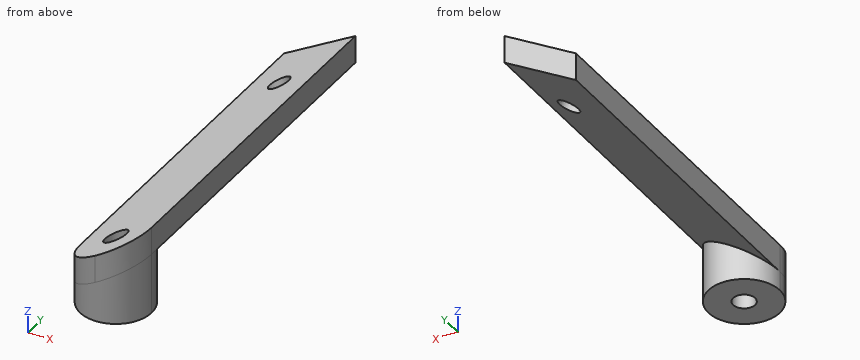
Autodesk Inventor part; units mm, degrees
ref_plane "YZ Plane" through (0, 0, 0) normal (1, 0, 0) x (0, 1, 0)
ref_plane "XZ Plane" through (0, 0, 0) normal (0, 1, 0) x (-1, 0, 0)
ref_plane "XY Plane" through (0, 0, 0) normal (0, 0, 1) x (1, 0, 0)
sketch "Sketch1" plane through (0, 0, 0) normal (0, 1, 0) x (-1, 0, 0)
  line L0 (0, 14.6647) -> (-13, 22.1703)
  line L1 (0, 14.6647) -> (15.0111, 14.6647) construction
  line L2 (-13, 22.1703) -> (-13, 27.1703)
  line L3 (0, 19.6647) -> (0, 14.6647)
  line L4 (0, 0) -> (-28.4468, 0) construction
  line L5 (-13, -7.1591) -> (0, -14.6647)
  line L6 (0, -14.6647) -> (0, -19.6647)
  line L7 (-13, 27.1703) -> (0, 27.1703)
  line L8 (0, 27.1703) -> (0, 19.6647)
  line L9 (0, -19.6647) -> (-13, -19.6647)
  line L10 (-13, -19.6647) -> (-13, -7.1591)
  point P0 (0, -12.7)
  dimension "d1" = 150
  dimension "d2" = 5
  dimension "d5" = 25.4
  dimension "d6" = 0
  dimension "d7" = 0
  dimension "d8" = 14.6647
  dimension "d9" = 13
  dimension "d10" = 13
  dimension "d11" = 5
extrude "Extrusion1" add sketch "Sketch1" against normal blind 70.4
fillet "Fillet1" radius 6.5 4 edges at (0, -70.4, 20.9175) (13, -70.4, 24.6703) (13, -70.4, -13.4119) (0, -70.4, -17.1647)
sketch "Sketch2" plane through (0, 0, 27.1703) normal (0, 0, 1) x (1, 0, 0)
  arc A0 (0, -63.9) -> (13, -63.9) centre (6.5, -63.9) ccw
  line L0 (0, -63.9) -> (0, 0)
  line L1 (0, 0) -> (13, 0)
  line L2 (13, 0) -> (13, -63.9)
  circle A1 centre (6.5, -63.9) radius 6.5
extrude "Extrusion2" add sketch "Sketch2" against normal blind 16 contours A1 A0
sketch "Sketch3" plane through (13, 0, -19.6647) normal (0, 0, -1) x (-1, 0, 0)
  arc A0 (0, -63.9) -> (13, -63.9) centre (6.5, -63.9) ccw
  line L0 (0, -63.9) -> (0, 0)
  line L1 (0, 0) -> (13, 0)
  line L2 (13, 0) -> (13, -63.9)
  circle A1 centre (6.5, -63.9) radius 6.5
extrude "Extrusion3" add sketch "Sketch3" against normal blind 16 contours A1 A0
sketch "Sketch4" plane through (0, 0, 0) normal (0, 1, 0) x (1, 0, 0)
  line L0 (0, -14.6647) -> (13, -22.1703)
  line L1 (13, -22.1703) -> (13, -27.1703)
  line L2 (13, -27.1703) -> (0, -27.1703)
  line L3 (0, -27.1703) -> (0, -14.6647)
  line L4 (13, 7.1591) -> (0, 14.6647)
  line L5 (0, 14.6647) -> (0, 19.6647)
  line L6 (0, 19.6647) -> (13, 19.6647)
  line L7 (13, 19.6647) -> (13, 7.1591)
  line L8 (13, -27.1703) -> (0, -19.6647)
  line L9 (13, -27.1703) -> (28.0111, -27.1703) construction
  line L10 (0, 19.6647) -> (13, 12.1591)
  point P0 (0, 0)
  dimension "d19" = 150
extrude "Extrusion4" cut sketch "Sketch4" against normal through all contours L8 L2 L3 | L10 L6 L7
sketch "Sketch5" plane through (13, -63.9, 27.1703) normal (-0.5, 0, 0.8660254) x (0.8660254, 0, 0.5)
  ellipse E0 centre (-7.5056, 0) end of major axis (-15.0111, 0) minor radius 6.5 (-15.0111, 0) -> (0, 0) ccw
  line L0 (-15.0111, 0) -> (-15.0111, 63.9)
  line L1 (-15.0111, 63.9) -> (0, 63.9)
  line L2 (0, 63.9) -> (0, 0)
  circle A0 centre (-7.5056, 51.2) radius 2
  point P0 (-24.8435, 63.9)
  dimension "d22" = 4
  dimension "d23" = 12.7
extrude "Extrusion5" cut sketch "Sketch5" against normal up to next contours A0
sketch "Sketch6" plane through (0, -63.9, -19.6647) normal (0.5, 0, -0.8660254) x (-0.8660254, 0, -0.5)
  ellipse E0 centre (-7.5056, 0) end of major axis (-15.0111, 0) minor radius 6.5 (-15.0111, 0) -> (0, 0) ccw
  line L0 (-15.0111, 0) -> (-15.0111, 63.9)
  line L1 (-15.0111, 63.9) -> (0, 63.9)
  line L2 (0, 63.9) -> (0, 0)
  circle A0 centre (-7.5056, 51.2) radius 2
  point P0 (-9.8323, 63.9)
  dimension "d26" = 4
  dimension "d27" = 12.7
extrude "Extrusion6" cut sketch "Sketch6" against normal up to next contours A0
sketch "Sketch7" plane through (6.5, -63.9, -3.6647) normal (0, 0, 1) x (1, 0, 0)
  circle A0 centre (0, 0) radius 6.5
  circle A1 centre (0, 0) radius 2
  point P0 (-6.5, 63.9)
  dimension "d30" = 4
extrude "Extrusion7" cut sketch "Sketch7" along normal through all both and the other way through all contours A1
sketch "Sketch9" plane through (0, 0, 0) normal (0, 1, 0) x (1, 0, 0)
  line L0 (-2.3389, 1.3365) -> (18.6443, 1.3365)
  line L1 (18.6443, 1.3365) -> (18.6443, 23.2553)
  line L2 (18.6443, 23.2553) -> (-2.3389, 23.2553)
  line L3 (-2.3389, 23.2553) -> (-2.3389, 1.3365)
  point P0 (0, 0)
extrude "Extrusion8" cut sketch "Sketch9" against normal through all
properties part number "terminal_mount"
Source: CAD feature listing. Evaluate the final solid. Frame: model axes, mm. Round coordinates to 2 decimals unless told otherwise and drop trailing zeros. Loops run counter-clockwise (first coordinate to the right, second up) from the corner with the lowest first, then second, coordinate; pieces in that order, holes last. Notation, with made-up numbers: M 34,-18.75 L 44,-18.75 A21 cw 44,11.25 Z; hole C 71,33.5 d1. An arc over 180 degrees is marked long. Use a Markdown table: item, result. Add a question column.
1. Ray query, line 1 along Y through (x, z) = (6.5, 16.25); line 2 along Y through (x, z) = (6.5, 19.75); line 3 along Y through (x, z) = (6.5, 19). Return the intervals inside material, ascending. Write a range as [from, to].
2. Cut plane D-D, the plane y = -9.5. Output: boundary loops of the cut face in (x, z).
3. Cut plane A-A, the plane y = -63. Output: boundary loops of the cut face in (x, z).
4. Cut plane B-B, the plane x = 2.25. Output: boundary loops of the cut face in (y, z), and give its area (3 significant figures).
5. Cut plane C-C, the plane z = 17.75. Output: boundary loops of the cut face in (x, y).
6. Contact query for flat-ended pins moving along their axis: pin 1 (5 mm diameter, centred on x = 8, y = -53.5, fed in from -Z); pin 2 (5 mm diameter, centred on x = 9, y = -41.5, fed in from -Z); pin 3 (3.5 mm diameter, centred on x = 6.5, y = -63.9, fed in from +Z). Output: stop coordinate, or through.
Solution:
| question | item | result |
|---|---|---|
| 1 | line 1 | y = [-70.4, -65.9], [-61.9, -57.4] |
| 1 | line 2 | y = [-70.4, -65.9], [-61.9, -13.5], [-11.9, 0] |
| 1 | line 3 | y = [-70.4, -65.9], [-61.9, 0] |
| 2 | outline | M 0,14.66 L 13,22.17 L 13,27.17 L 0,19.66 Z |
| 3 | outline | M 0,14.66 L 0.06,14.7 L 0.06,11.17 L 4.71,11.17 L 4.71,22.39 L 0,19.66 Z; M 8.29,11.17 L 12.94,11.17 L 12.94,22.13 L 13,22.17 L 13,27.17 L 8.29,24.45 Z |
| 4 | outline | M -68.82,11.17 L -58.98,11.17 L -58.98,15.96 L 0,15.96 L 0,20.96 L -68.82,20.96 Z |
| 4 | area | 391 mm2 |
| 5 | outline | M 0,-63.9 A6.5 ccw 5.34,-70.3 A6.5 ccw long 5.34,-57.5 L 5.34,0 L 0,0 Z; hole C 6.5,-63.9 d4 |
| 6 | pin 1 | stops at z = 17.84 |
| 6 | pin 2 | stops at z = 18.42 |
| 6 | pin 3 | passes through |
